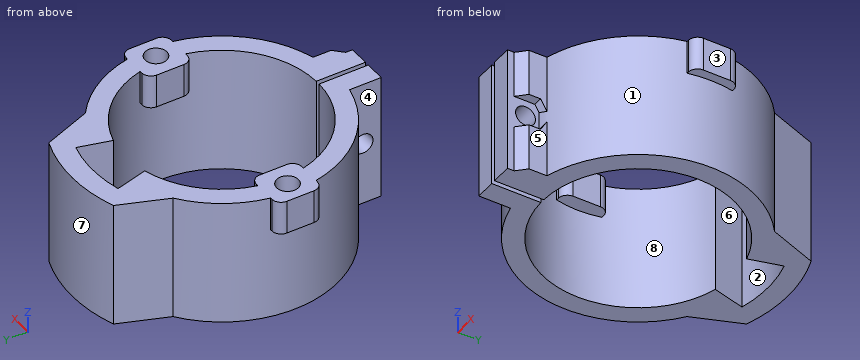
Autodesk Inventor part; units mm, degrees
ref_plane "YZ Plane" through (0, 0, 0) normal (1, 0, 0) x (0, 1, 0)
ref_plane "XZ Plane" through (0, 0, 0) normal (0, 1, 0) x (-1, 0, 0)
ref_plane "XY Plane" through (0, 0, 0) normal (0, 0, 1) x (1, 0, 0)
sketch "スケッチ1" plane through (0, 0, 0) normal (0, 0, 1) x (1, 0, 0)
  line L0 (0, 0) -> (10, 0)
  line L1 (10, 0) -> (10, 32.05)
  line L2 (10, 32.05) -> (0, 32.05)
  line L3 (0, 32.05) -> (0, 0)
  circle A0 centre (5, 32.05) radius 25.55
  arc A1 (16.3038, 63.1068) -> (-6.3038, 63.1068) centre (5, 32.05) ccw
  line L4 (5, 32.05) -> (16.3038, 63.1068) construction
  line L5 (5, 32.05) -> (-6.3038, 63.1068) construction
  line L6 (-6.3038, 63.1068) -> (-3.7386, 56.0591)
  line L7 (16.3038, 63.1068) -> (13.7386, 56.0591)
  arc A2 (12.3893, 59.6272) -> (-2.3893, 59.6272) centre (5, 32.05) ccw
  arc A3 (10.4481, 52.3827) -> (-0.4481, 52.3827) centre (5, 32.05) ccw
  line L8 (-2.3893, 59.6272) -> (-0.4481, 52.3827)
  line L9 (12.3893, 59.6272) -> (10.4481, 52.3827)
  point P0 (0, 6.994)
  point P1 (10, 6.994)
  point P2 (5, 65.1)
  point P3 (5, 60.6)
  dimension "d0" = 32.05
  dimension "d1" = 51.1
  dimension "d27" = 10
  dimension "d28" = 5
  dimension "d43" = 21.05
  dimension "d44" = 7.5
  dimension "d45" = 4.5
  dimension "d46" = 30
  dimension "d47" = 5
extrude "押し出し1" add sketch "スケッチ1" along normal blind 28 contours L3 A0 L1 L0 | A0 L8 A3 L9 L1 L2 L3 | L3 L2 L1 A0 | L6 A1 L7 A0 L9 A2 L8
sketch "スケッチ2" plane through (0, 0, 28) normal (0, 0, 1) x (1, 0, 0)
  arc A0 (10, 6.994) -> (0, 6.994) centre (5, 32.05) ccw
  point P0 (0, 0)
hole "穴1" at (5, 32.05, 28) direction (0, 0, -1) diameter 42.4 end through all
sketch "スケッチ3" plane through (0, 0, 28) normal (0, 0, 1) x (1, 0, 0)
  line L0 (0, 0) -> (10, 0)
  line L1 (4.5, 0) -> (5.5, 0)
  line L2 (5.5, 0) -> (5.5, 32.05)
  line L3 (5.5, 32.05) -> (4.5, 32.05)
  line L4 (4.5, 32.05) -> (4.5, 0)
  line L5 (0, 6.994) -> (0, 0)
  arc A0 (-0.487, 52.5276) -> (10.487, 52.5276) centre (5, 32.05) ccw
  point P0 (5, 0)
  point P1 (5, 0)
  dimension "d14" = 1
extrude "押し出し2" cut sketch "スケッチ3" against normal up to surface (28 mm away)
sketch "スケッチ4" plane through (10, 0, 0) normal (1, 0, 0) x (0, 0, -1)
  circle A0 centre (-14, 4) radius 1.5
  line L0 (0, 0) -> (-28, 0)
  line L1 (0, 0) -> (0, 6.994)
  line L2 (-14, 0) -> (-14, 10)
  point P0 (0, 10)
  dimension "d17" = 4
  dimension "d19" = 3
hole "穴2" at (10, 4, 14) direction (-1, 0, 0) diameter 4.4 end through all
sketch "スケッチ7" plane through (10, 0, 0) normal (1, 0, 0) x (0, 0, -1)
  circle A0 centre (-14, 4) radius 2.2
  line L0 (-14, 8.1569) -> (-10.4, 6.0785)
  line L1 (-10.4, 6.0785) -> (-10.4, 1.9215)
  line L2 (-10.4, 1.9215) -> (-14, -0.1569)
  line L3 (-14, -0.1569) -> (-17.6, 1.9215)
  line L4 (-17.6, 1.9215) -> (-17.6, 6.0785)
  line L5 (-17.6, 6.0785) -> (-14, 8.1569)
  line L6 (-28, 10.8559) -> (-28, 0)
  line L7 (0, 0) -> (0, 6.994)
  line L8 (-28, 10.8559) -> (0, 10.8559)
  line L9 (0, 10.8559) -> (0, 3.497)
  line L10 (0, 3.497) -> (-28, 3.497)
  line L11 (-28, 3.497) -> (-28, 10.8559)
  point P0 (-10.4, 3.497)
  point P1 (-28, 3.497)
  point P2 (-17.6, 3.497)
  dimension "d35" = 7.2
extrude "押し出し5" add sketch "スケッチ7" along normal blind 2 contours L10 L6 L8 L9 L7 L1 L0 L5 L4
chamfer "面取り1" distance 2 angle 45 2 edges at (10, 3.497, 22.8) (10, 3.497, 5.2)
chamfer "面取り2" distance 7.5 angle 45 2 edges at (-3.7386, 56.0591, 14) (13.7386, 56.0591, 14)
sketch "スケッチ8" plane through (0, 0, 28) normal (0, 0, 1) x (1, 0, 0)
  arc A0 (12, 7.4776) -> (20.3335, 52.4874) centre (5, 32.05) ccw
  line L0 (30.056, 37.05) -> (32.5, 37.05)
  line L1 (32.5, 37.05) -> (32.5, 27.05)
  line L2 (32.5, 27.05) -> (30.056, 27.05)
  line L3 (30.056, 27.05) -> (30.056, 37.05)
  arc A1 (-10.3335, 52.4874) -> (0, 6.994) centre (5, 32.05) ccw
  line L4 (-20.056, 37.05) -> (-22.5, 37.05)
  line L5 (-22.5, 37.05) -> (-22.5, 27.05)
  line L6 (-22.5, 27.05) -> (-20.056, 27.05)
  line L7 (-20.056, 27.05) -> (-20.056, 37.05)
  arc A2 (-10.3335, 52.4874) -> (0, 6.994) centre (5, 32.05) ccw
  line L8 (30.056, 37.05) -> (23.0125, 37.05)
  line L9 (23.0125, 37.05) -> (23.0125, 27.05)
  line L10 (23.0125, 27.05) -> (30.056, 27.05)
  line L11 (30.056, 27.05) -> (30.056, 37.05)
  line L12 (-20.056, 37.05) -> (-13.0125, 37.05)
  line L13 (-13.0125, 37.05) -> (-13.0125, 27.05)
  line L14 (-13.0125, 27.05) -> (-20.056, 27.05)
  line L15 (-20.056, 27.05) -> (-20.056, 37.05)
  arc A3 (12, 7.4776) -> (20.3335, 52.4874) centre (5, 32.05) ccw
  point P0 (0, 0)
  dimension "d51" = 55
  dimension "d52" = 10
  dimension "d57" = 36.025
extrude "押し出し6" add sketch "スケッチ8" against normal blind 7.5
sketch "スケッチ9" plane through (0, 0, 28) normal (0, 0, 1) x (1, 0, 0)
  line L0 (32.5, 27.05) -> (32.5, 37.05)
  arc A0 (5.5, 10.8559) -> (10.487, 52.5276) centre (5, 32.05) ccw
  point P0 (0, 0)
  point P1 (-18.0125, 32.05)
  point P2 (28.0125, 32.05)
  point P3 (32.5, 32.05)
  dimension "d55" = 46.025
  dimension "d56" = 23.0125
hole "穴3" at (-18.0125, 32.05, 28) at (28.0125, 32.05, 28) direction (0, 0, -1) diameter 4.8 depth 5
fillet "フィレット1" radius 2 8 edges at (-22.5, 37.05, 24.25) (-22.5, 27.05, 24.25) (-13.0125, 37.05, 24.25) (-13.0125, 27.05, 24.25) (32.5, 37.05, 24.25) (32.5, 27.05, 24.25) (23.0125, 37.05, 24.25) (23.0125, 27.05, 24.25)
equation "\"d28\" = 0.5 * d27"
properties part number "軸止め" material "ABS プラスチック"
Can you work these out from the model? Positions are in its coordinate system, mm. Face numbers are marked on the shaded views. A direction names the side the tool comes from. Coordinates: 2 decimals unless noted, no trailing zeros. Write each loop counter-clockwise with the first axis right and the second up, starting at its lowest first coordinate (ties: lowest second). Pieces come first, ordered by that corner, then holes. Notation, with made-up numbers: (14.25, 49) -> (19.25, 49) arc R27 ccw to (19.25, 77) -> close; hole circle Ø3 at (58, 18.25). An arc over 180 degrees is marked (long way). Write item = value, one per line.
(1) Imagine slicing it at A-A (y = 32.05). Please give me the cut outline in (x, z).
Verdict:
outline = (-22.5, 20.5) -> (-20.55, 20.5) -> (-20.55, 0) -> (-16.2, 0) -> (-16.2, 20.5) -> (-13.01, 20.5) -> (-13.01, 28) -> (-15.61, 28) -> (-15.61, 23) -> (-20.41, 23) -> (-20.41, 28) -> (-22.5, 28) -> close; (23.01, 20.5) -> (26.2, 20.5) -> (26.2, 0) -> (30.55, 0) -> (30.55, 20.5) -> (32.5, 20.5) -> (32.5, 28) -> (30.41, 28) -> (30.41, 23) -> (25.61, 23) -> (25.61, 28) -> (23.01, 28) -> close
(2) Imagine slicing it at D-D (y = 23). Please give me the cut outline in (x, z).
Verdict:
outline = (-18.89, 0) -> (-14.17, 0) -> (-14.17, 28) -> (-18.89, 28) -> close; (24.17, 0) -> (28.89, 0) -> (28.89, 28) -> (24.17, 28) -> close
(3) Imagine slicing it at C-C (z = 14). State how many separate pieces and enclosed holes the cut face has, and give its area (3 significant figures).
Verdict:
separate_pieces = 3
enclosed_holes = 0
area = 766 mm^2
(4) For pin 1 (3.5 mm diameter, centred on x = -15, y = 32.5, fed in from -Z); pin 2 (10 mm diameter, centred on y = 14.5, z = 22.5, fed in from +X); pin 3 (2 mm diameter, centred on y = 8, z = 3, fed in from -X); pin 4 (1.5 mm diameter, centred on x = -2, z = 25, fed in from +Y), each with a flat end and sliding along its axis, tell me the tip position at first contact or that it passes through.
Verdict:
pin_1 = 0
pin_2 = 27.26
pin_3 = -6.02
pin_4 = 64.5
(5) If I drill on probe 1 along X at (y, z) = (32.05, 24.35); probe 2 along Z at (x, y) = (1.05, 4); probe 3 along X at (y, z) = (31.5, 1.5), over which ranges is the centre line in solid material (lowest first)?
Verdict:
probe_1 = -22.5 to -20.41, -15.61 to -13.01, 23.01 to 25.61, 30.41 to 32.5
probe_2 = 0 to 11.8, 16.2 to 28
probe_3 = -20.54 to -16.19, 26.19 to 30.54
(6) Imagine slicing it at B-B (x = -8). Please give me the cut outline in (y, z).
Verdict:
outline = (10.05, 0) -> (15.3, 0) -> (15.3, 28) -> (10.05, 28) -> close; (48.8, 0) -> (58.64, 0) -> (58.64, 28) -> (48.8, 28) -> close
(7) Thinking about a two-plate mould opening in Y: for the marked faces 1, 2 and 3, which applies, +Y half, -Y half, draft (parallel to the pull), parting line (faces both ways), or undercut?
Verdict:
face_1 = parting line
face_2 = undercut
face_3 = draft
(8) On a 3-axis mill with a long thin cutter (end or side, diameter ignored), from which of +Z, -Z, +X, -X, +Y, -Y can I reach the whole of each face in a straight line? I mean the marked faces 4, 5, 6, 7 and 8. Say none if no direction works.
Verdict:
face_4 = +Z, -Z, -X, -Y
face_5 = +Z, -Z, +X, -Y
face_6 = +Z, -Z
face_7 = +Z, -Z, +Y
face_8 = -Z
